```python
from build123d import *

# Parameters (mm, degrees)
SKETCH_1_R          = 4.5
SKETCH_1_R_2        = 3.5
EXTRUDE_1_DEPTH     = 5
SKETCH_2_R          = 15
EXTRUDE_2_DEPTH     = 3
SKETCH_3_R          = 2
CUT_EXTRUDE_1_DEPTH = 3
SKETCH_4_R          = 1.5
CUT_EXTRUDE_2_DEPTH = 3


with BuildPart() as part:
    # 草图1 → 凸台-拉伸1 (new body)
    with BuildSketch(Plane.XY):
        Circle(SKETCH_1_R)
        Circle(SKETCH_1_R_2, mode=Mode.SUBTRACT)
    extrude(amount=EXTRUDE_1_DEPTH)

    # 草图2 → 凸台-拉伸2 (add)
    with BuildSketch(Plane.XY.offset(5)):
        Circle(SKETCH_2_R)
    extrude(amount=EXTRUDE_2_DEPTH)

    # 草图3 → 切除-拉伸1 (cut)
    with BuildSketch(Plane.XY.offset(8)):
        with Locations((-10, 0)):
            Circle(SKETCH_3_R)
        with Locations((10, 0)):
            Circle(SKETCH_3_R)
        with Locations((0, 10)):
            Circle(SKETCH_3_R)
        with Locations((0, -10)):
            Circle(SKETCH_3_R)
    extrude(amount=-CUT_EXTRUDE_1_DEPTH, mode=Mode.SUBTRACT)

    # 草图4 → 切除-拉伸2 (cut)
    with BuildSketch(Plane.XY.offset(8)):
        Circle(SKETCH_4_R)
    extrude(amount=-CUT_EXTRUDE_2_DEPTH, mode=Mode.SUBTRACT)


solid = part.part
```
Could you check a few things on this model? Use its own coordinates, in mm. A direction names the side the tool comes from. Coordinates: 2 decimals unless noted, no trailing zeros. Write each loop counter-clockwise with the first axis right and the second up, starting at its lowest first coordinate (ties: lowest second). Pieces come first, ordered by that corner, then holes. Notation, with made-up numbers: (30, -31.5) -> (39, -31.5) arc R34 cw to (39, -1.5) -> close; hole circle Ø2 at (28.5, -37). An arc over 180 degrees is marked (long way). One line per question, with ' | ' between items. Start each with the question number.
1. Thinking about a two-plate mould opening in X: for faces 3 (the face through (0, -4, 0)), 4 (the face through (3.233, -1.341, 2.465)), 5 (the face through (-0.59, 4.46, 2.46)), 6 (the face through (-11.6, -1.2, 6.5)), which applies, pulls with the +X half, pulls with the -X half, needs draft (parallel to the pull), parting line crosses it, or undercut?
2. Will these pins go through, and if not, where does the flat tip stop? P1, Ø5, axis at x = 0, y = -10, coming from the +Z side; P2, Ø2, axis at x = -5.5, y = -6, coming from the -Z side; P3, Ø1, axis at x = -9.5, z = 6, coming from the +Y side; P4, Ø3.5, axis at x = 10, y = 0, coming from the -Z side.
3. For faces 1 (the face through (0, -8, 7)), 2 (the face through (3, 4, 5)), which set-ups out of +Z, -Z, +X, -X, +Y, -Y let a thin tool reach every point of the face, with its end or its side?
4. Please list where these lines run through material, in increasing order: line 1 along Y through (x, z) = (0, 5.7); line 2 along Z through (x, y) = (-2.25, -0.5); line 3 along Y through (x, z) = (0, 1.25).
5. If we section it at A-A (y = 0): Please give me the cut outline in (x, z), and give its area (3 significant figures).
6. If we section it at D-D (y = -10): Please give me the cut outline in (x, z), and give its area (3 significant figures).
7. If we section it at C-C (z = 7): Please give me the cut outline in (x, y).
Return value:
1) face 3: needs draft | face 4: undercut | face 5: parting line crosses it | face 6: undercut
2) P1: stops at z = 8 | P2: stops at z = 5 | P3: stops at y = 12 | P4: passes through
3) face 1: +Z, -Z | face 2: -Z
4) line 1: y = -15 to -12, -8 to -1.5, 1.5 to 8, 12 to 15 | line 2: z = 5 to 8 | line 3: y = -4.5 to -3.5, 3.5 to 4.5
5) outline: (-15, 5) -> (-12, 5) -> (-12, 8) -> (-15, 8) -> close; (-8, 5) -> (-4.5, 5) -> (-4.5, 0) -> (-3.5, 0) -> (-3.5, 5) -> (-1.5, 5) -> (-1.5, 8) -> (-8, 8) -> close; (1.5, 5) -> (3.5, 5) -> (3.5, 0) -> (4.5, 0) -> (4.5, 5) -> (8, 5) -> (8, 8) -> (1.5, 8) -> close; (12, 5) -> (15, 5) -> (15, 8) -> (12, 8) -> close | area: 67.0 mm²
6) outline: (-11.18, 5) -> (-2, 5) -> (-2, 8) -> (-11.18, 8) -> close; (2, 5) -> (11.18, 5) -> (11.18, 8) -> (2, 8) -> close | area: 55.1 mm²
7) outline: circle Ø30 at (0, 0); hole circle Ø4 at (-10, 0); hole circle Ø4 at (0, -10); hole circle Ø4 at (0, 10); hole circle Ø3 at (0, 0); hole circle Ø4 at (10, 0)
